For this review, take the finished solid that the model builds, in its own axes (mm). A direction names the side the tool comes from. Coordinates: 2 decimals unless noted, no trailing zeros. Order: outer loops, then holes, each group sorted by start corner. A loop starts at its lowest first (then second) coordinate and runs counter-clockwise, first axis right, second up. Notation, with made-up numbers: (-39, -36) -> (17, -36) arc R12 cw to (17, -28) -> close; hole circle Ø4 at (-15, -33.5). An arc over 180 degrees is marked (long way). Write item = value, one per line. Start each with the question number.
1) Consider section A-A on z = 3. Give the boundary of the cut face in (x, y) (3 decimals).
2) Wall thickness on probe 1 along X at (y, z) = (1, 2.5) (3 decimals); probe 2 along X at (y, z) = (-15, 19) (3 decimals); probe 3 along Y at (x, z) = (33.5, 57.5): over which ranges is each line inside the solid? List them lowest first. Write a range as [from, to].
3) Insertion check: pin 1 Ø14 at (y, z) = (-16.5, 22.5) entering from -X (3 decimals); pin 2 Ø15.5 at (x, z) = (60.5, 38) entering from +Y; pin 3 Ø5 at (y, z) = (-22.5, 39) entering from -X. Each pin has a flat end and moves straight along its axis. Give the tip position at first contact, or say it passes through.
4) Consider section B-B on y = -44.5. Give the boundary of the cut face in (x, z) (3 decimals), and give its area (3 significant figures).
5) Machinability: for faces 1 (the face through (61, 2, 61.925)), 2 (the face through (47, -25.4, 42)), 3 (the face through (45.8, -0.4, 38.1)), which of the approach directions +Z, -Z, +X, -X, +Y, -Y give a long, thin tool a straight path to every point of the face, cutting with its end or side? Answer none if there is none.
from build123d import *

# Parameters (mm, degrees)
F1_DEPTH = 63.5
F2_DEPTH = 25.4
F3_DEPTH = 7.9375
F0_W     = 25.9641238877
F0_H     = 19.05
F4_DEPTH = 25.4
F6_R     = 6.35


with BuildPart() as f1:
    # F0 (on Front) → F1 (new body, symmetric)
    with BuildSketch(Plane.XZ):
        Polygon((22.225, 9.525), (-41.275, 9.525), (-41.275, -9.525), (41.275, -9.525), (41.275, 9.525), align=None)
    extrude(amount=F1_DEPTH, both=True)

    # F0 (on Front) → F2 (join, symmetric)
    with BuildSketch(Plane.XZ):
        with BuildLine():
            Line((22.225, 27.0002), (22.225, 9.525))
            Line((22.225, 9.525), (41.275, 9.525))
            Line((41.275, 9.525), (41.275, 27.0002))
            ThreePointArc((41.275, 27.0002), (45.9246798487, 38.2255201513), (57.15, 42.8752))
            Line((57.15, 42.8752), (60.325, 42.8752))
            Line((60.325, 42.8752), (60.325, 61.9252))
            Line((60.325, 61.9252), (57.15, 61.9252))
            add(Edge.make_bspline(
                [(55.8373775892, 61.9005244599), (56.2776364161, 61.9107392271), (56.7152170121, 61.9189622944), (57.15, 61.9252)],
                knots=[110.241102344, 110.241102344, 110.241102344, 110.241102344, 111.5045361635, 111.5045361635, 111.5045361635, 111.5045361635], degree=3))
            ThreePointArc((55.8373775892, 61.9005244599), (31.9944940152, 51.2273777896), (22.225, 27.0002))
        make_face()
    extrude(amount=F2_DEPTH, both=True)

    # F0 (on Front) → F3 (join, symmetric)
    with BuildSketch(Plane.XZ):
        with BuildLine():
            add(Edge.make_bspline(
                [(-41.275, 9.525), (-41.3829236444, 44.9542144396), (17.4225293824, 61.0092334589), (55.8373775892, 61.9005244599)],
                knots=[0, 0, 0, 0, 110.241102344, 110.241102344, 110.241102344, 110.241102344], degree=3))
            Line((-41.275, 9.525), (22.225, 9.525))
            Line((22.225, 9.525), (22.225, 27.0002))
            ThreePointArc((22.225, 27.0002), (31.9944940152, 51.2273777896), (55.8373775892, 61.9005244599))
        make_face()
    extrude(amount=F3_DEPTH, both=True)

    # F0 (on Front) → F4 (join, symmetric)
    with BuildSketch(Plane.XZ):
        with Locations((73.3070619439, 52.4002)):
            Rectangle(F0_W, F0_H)
    extrude(amount=F4_DEPTH, both=True)

    # F0 (on Front) → F5 (revolve)
    with BuildSketch(Plane.XZ):
        Polygon((86.2891238877, 66.675), (86.2891238877, 61.9252), (86.2891238877, 42.8752), (86.2891238877, 38.1), (111.125, 38.1), (111.125, 66.675), align=None)
    revolve(axis=Axis((86.2891238877, 0, 50.0126), (0, 0, 1)))

    # F6
    f6_edges = [f1.edges().sort_by_distance(p)[0] for p in [
        (41.275, 63.5, 0),
        (-41.275, 63.5, 0),
        (-41.275, -63.5, 0),
        (41.275, -63.5, 0),
    ]]
    fillet(f6_edges, radius=F6_R)


solid = f1.part
Answer sheet:
q1.outline = (-41.275, -57.15) arc R6.35 ccw to (-34.925, -63.5) -> (34.925, -63.5) arc R6.35 ccw to (41.275, -57.15) -> (41.275, 57.15) arc R6.35 ccw to (34.925, 63.5) -> (-34.925, 63.5) arc R6.35 ccw to (-41.275, 57.15) -> close
q2.probe_1 = [-41.275, 41.275]
q2.probe_2 = [22.225, 41.275]
q2.probe_3 = [-7.94, 7.94]
q3.pin_1 = 22.225
q3.pin_2 = 25.4
q3.pin_3 = 23.54
q4.outline = (-41.275, -9.525) -> (41.275, -9.525) -> (41.275, 9.525) -> (-41.275, 9.525) -> close
q4.area = 1,570 mm2
q5.face_1 = +Z, -X
q5.face_2 = +Z, +X, -X, -Y
q5.face_3 = -Z, +Y, -Y
